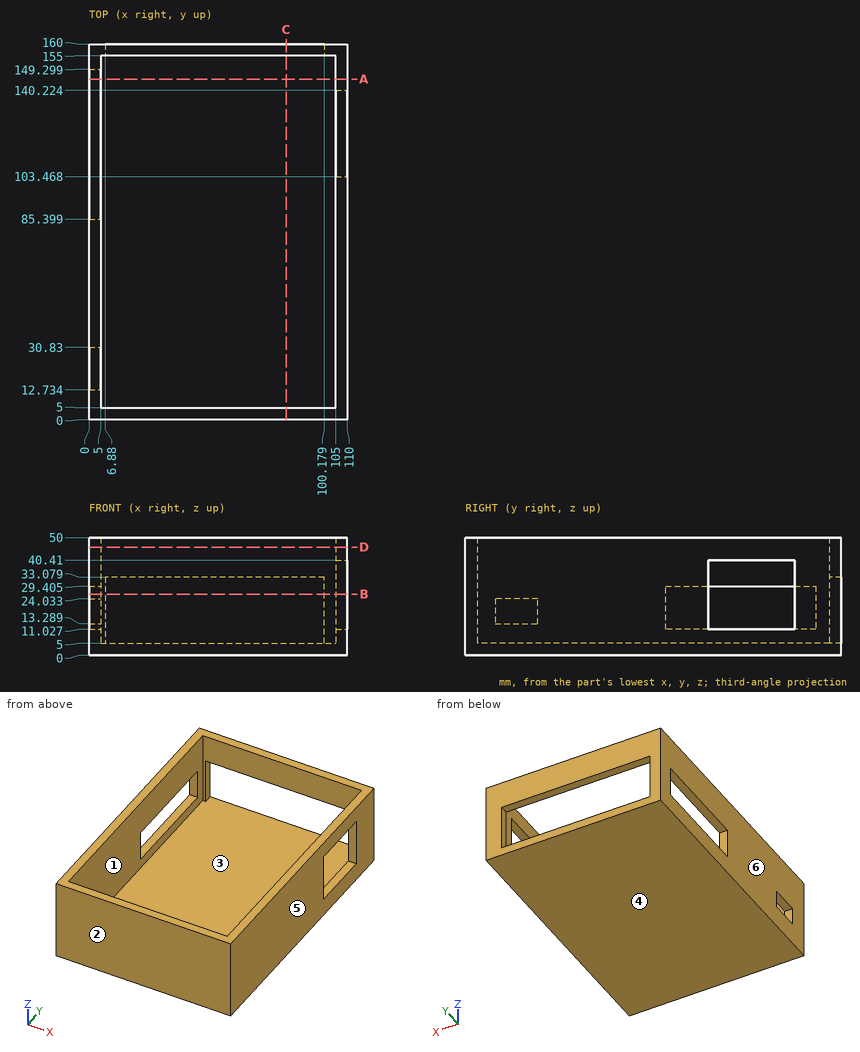
Verification items for this drawing (mm, ordinates from the low corner). A direction names the side the tool comes from. Give positions to 0.01 mm unless a question says otherwise; leave off trailing zeros. Loops run counter-clockwise (first coordinate to the right, second up) from the corner with the lowest first, then second, coordinate; pieces in that order, holes last. Notation, with made-up numbers: M 60,-32.5 L 94,-32.5 A24 cw 94,-21.5 Z; hole C 4,59.5 d5. An arc over 180 degrees is marked long. Write item = value, one per line.
(1) Sectioned sample at A-A, the plane y = 145. Record the cut outline in (x, z) (1 decimal), plus the area to 3 significant figures.
Answer below:
outline = M 0,0 L 110,0 L 110,50 L 105,50 L 105,5 L 5,5 L 5,11 L 0,11 Z; M 0,29.4 L 5,29.4 L 5,50 L 0,50 Z
area = 908 mm2
(2) Tool access check on the marked faces 1 and 2. Record the directions out of +Z, -Z, +X, -X, +Y, -Y that give a thin tool (end or side, any length) a straight path to the whole face; none if there is none.
Answer below:
face_1 = +Z
face_2 = +Z, -Z, +X, -X, -Y
(3) Gauge pin test, flat ends, axial feed: pin 1 Ø1.5 at (x, y) = (2.5, 22.5) entering from -Z; pin 2 Ø3 at (x, y) = (85, 16.5) entering from +Z; pin 3 Ø1.5 at (x, z) = (13.5, 18) entering from +Y. Record the tip position at first contact, or that the pin passes through.
Answer below:
pin_1 = 0
pin_2 = 5
pin_3 = 5
(4) Sectioned sample at C-C, the plane x = 84. Record the cut outline in (y, z).
Answer below:
outline = M 0,0 L 160,0 L 160,5 L 5,5 L 5,50 L 0,50 Z; M 155,33.08 L 160,33.08 L 160,50 L 155,50 Z
(5) Release check for a two-part mould opening along X. For the marked faces 3, 4, 5 and 6 record: released by +X, released by -X, zero draft, split by the parting line, or undercut.
Answer below:
face_3 = undercut
face_4 = zero draft
face_5 = released by +X
face_6 = released by -X
(6) Sectioned sample at D-D, the plane z = 46. Record the cut outline in (x, y).
Answer below:
outline = M 0,0 L 110,0 L 110,160 L 0,160 Z; hole M 5,5 L 105,5 L 105,155 L 5,155 Z
(7) Sectioned sample at B-B, the plane z = 26. Record the cut outline in (x, y) (1 decimal), plus the area to 3 significant figures.
Answer below:
outline = M 0,0 L 110,0 L 110,103.5 L 105,103.5 L 105,5 L 5,5 L 5,85.4 L 0,85.4 Z; M 0,149.3 L 5,149.3 L 5,155 L 6.9,155 L 6.9,160 L 0,160 Z; M 100.2,155 L 105,155 L 105,140.2 L 110,140.2 L 110,160 L 100.2,160 Z
area = 1,630 mm2
(8) Material ranges on line 1 (Y direction, x = 101.5, z = 45.5); line 2 (Z direction, x = 105.5, y = 126.5); line 3 (X direction, y = 36, z = 13), recorded low to high. Write a range as [from, to].
Answer below:
line_1 = [0, 5], [155, 160]
line_2 = [0, 11.03], [40.41, 50]
line_3 = [0, 5], [105, 110]
